from build123d import *

# Parameters (mm, degrees)
SKETCH1_R           = 66.9925
SKETCH1_R_2         = 63.8175
BOSS_EXTRUDE1_DEPTH = 12.7
CUT_EXTRUDE1_START  = -66.9925
SKETCH2_R           = 1.5875
CUT_EXTRUDE1_DEPTH  = 3.194748
CIRPATTERN1_COUNT   = 4
CHAMFER1_SIZE       = 1.27


with BuildPart() as part:
    # Sketch1 → Boss-Extrude1 (new body)
    with BuildSketch(Plane(origin=(0, 0, 0), x_dir=(1, 0, 0), z_dir=(0, 1, 0))):
        Circle(SKETCH1_R)
        Circle(SKETCH1_R_2, mode=Mode.SUBTRACT)
    extrude(amount=BOSS_EXTRUDE1_DEPTH)

    # Sketch2 → Cut-Extrude1 (cut)
    with BuildSketch(Plane.XY.offset(CUT_EXTRUDE1_START)):
        with Locations((0, 6.35)):
            Circle(SKETCH2_R)
    cut_extrude1 = extrude(amount=CUT_EXTRUDE1_DEPTH, mode=Mode.SUBTRACT)

    # CirPattern1: Cut-Extrude1 ×4 about axis
    cirpattern1_axis = Axis((0, 12.7, 0), (0, -1, 0))
    for i in range(1, CIRPATTERN1_COUNT):
        add(cut_extrude1.rotate(cirpattern1_axis, i * 360 / CIRPATTERN1_COUNT), mode=Mode.SUBTRACT)

    # Chamfer1
    chamfer1_edges = [part.edges().sort_by_distance(p)[0] for p in [
        (-63.8175, 0, 0),
    ]]
    chamfer(chamfer1_edges, length=CHAMFER1_SIZE)


solid = part.part
Work out the finished part from the listing and answer in its coordinate system (mm). Give positions to 0.01 mm unless a question says otherwise; leave off trailing zeros. Write each loop counter-clockwise with the first axis right and the second up, starting at its lowest first coordinate (ties: lowest second). Pieces come first, ordered by that corner, then holes.
Q1. The part is cut by section C-C on y = 6.35. Give the vertices of the cut face in (x, z) (1 decimal).
Answer:
outline: (-67, -1.6) arc R67 ccw to (-1.6, -67) - (-1.6, -63.8) arc R63.8 cw to (-63.8, -1.6) - close; (-67, 1.6) - (-63.8, 1.6) arc R63.8 cw to (-1.6, 63.8) - (-1.6, 67) arc R67 ccw to start; (1.6, -67) arc R67 ccw to (67, -1.6) - (63.8, -1.6) arc R63.8 cw to (1.6, -63.8) - close; (1.6, 63.8) arc R63.8 cw to (63.8, 1.6) - (67, 1.6) arc R67 ccw to (1.6, 67) - close
Q2. Straight lines are drawn through the part: L1, parallel to X at y = 4, z = 0; L2, parallel to Y at x = 66.2, z = 0; L3, parallel to X at y = 9.25, z = 21. For each, find the intervals that lie inside material, in ascending order.
Answer:
L1: x = -66.99 to -63.82, 63.82 to 66.99
L2: y = 0 to 4.76, 7.94 to 12.7
L3: x = -63.62 to -60.26, 60.26 to 63.62
Q3. For a pull along Y with two mould halves and no side action, classify faces 1 (the face through (24.5, 12.7, 59.2)), 2 (the face through (0.73, 4.94, -65.42)), 3 (the face through (65.42, 4.94, 0.73)), 4 (the face through (-10, 0, -65)) as released by +Y, released by -Y, zero draft, split by the parting line, or undercut.
Answer:
face 1: released by +Y
face 2: undercut
face 3: undercut
face 4: released by -Y
Q4. The part is cut by section A-A on x = 0. Give the vertices of the cut face in (y, z), and give its area (3 significant figures).
Answer:
outline: (0, -66.99) - (4.76, -66.99) - (4.76, -63.82) - (1.27, -63.82) - (0, -65.09) - close; (0, 65.09) - (1.27, 63.82) - (4.76, 63.82) - (4.76, 66.99) - (0, 66.99) - close; (7.94, -66.99) - (12.7, -66.99) - (12.7, -63.82) - (7.94, -63.82) - close; (7.94, 63.82) - (12.7, 63.82) - (12.7, 66.99) - (7.94, 66.99) - close
area: 58.9 mm2
Q5. The part is cut by section B-B on z = 0. Give the vertices of the cut face in (x, y).
Answer:
outline: (-66.99, 0) - (-65.09, 0) - (-63.82, 1.27) - (-63.82, 4.76) - (-66.99, 4.76) - close; (-66.99, 7.94) - (-63.82, 7.94) - (-63.82, 12.7) - (-66.99, 12.7) - close; (63.82, 1.27) - (65.09, 0) - (66.99, 0) - (66.99, 4.76) - (63.82, 4.76) - close; (63.82, 7.94) - (66.99, 7.94) - (66.99, 12.7) - (63.82, 12.7) - close
Q6. Given pin 1 (5 mm diameter, centred on y = 3.5, z = 44, fed in from -X); pin 2 (5 mm diameter, centred on y = 8.5, z = 52, fed in from +X); pin 3 (3 mm diameter, centred on x = -34, y = 5, fed in from +Z), each flat-ended and moving along its own axis, determine where each tip first touches the part or whether it passes through.
Answer:
pin 1: stops at x = -52.59
pin 2: stops at x = 45.14
pin 3: stops at z = 58.58
